from build123d import *

# Parameters (mm, degrees)
SKETCH_1_W           = 10
SKETCH_1_H           = 10
SKETCH_1_W_2         = 8
SKETCH_1_H_2         = 8
EXTRUDE_1_DEPTH      = 106.066
SKETCH_2_R           = 1
CUT_EXTRUDE_1_DEPTH  = 10
EXTRUDE_START        = -22
EXTRUDE_3_OUTLINE_R  = 1
EXTRUDE_3_DEPTH      = 34
EXTRUDE_7_DEPTH      = 15.36
EXTRUDE_7_DEPTH_BACK = 25.36
SKETCH_9_R           = 1
EXTRUDE_8_DEPTH      = 5
EXTRUDE_8_DEPTH_BACK = 15


# Read off the part's stored shape, not the designer's step: the extrude step
with BuildPart() as part:
    # Sketch 1 → Extrude 1 (new body)
    with BuildSketch(Plane.XY):
        with Locations((5, 5)):
            Rectangle(SKETCH_1_W, SKETCH_1_H)
        with Locations((5, 5)):
            Rectangle(SKETCH_1_W_2, SKETCH_1_H_2, mode=Mode.SUBTRACT)
    extrude(amount=EXTRUDE_1_DEPTH)

    # Sketch 2 → Cut-Extrude 1 (cut)
    with BuildSketch(Plane(origin=(10, 0, 0), x_dir=(0, 0, -1), z_dir=(1, 0, 0))):
        with Locations((-10, 5)):
            Circle(SKETCH_2_R)
    extrude(amount=-CUT_EXTRUDE_1_DEPTH, mode=Mode.SUBTRACT)

    # Extrude 3 outline → Extrude 3 (add)
    with BuildSketch(Plane(origin=(10, 0, 0), x_dir=(0, 0, -1), z_dir=(1, 0, 0)).offset(EXTRUDE_START)):
        with Locations((-10, 5)):
            Circle(EXTRUDE_3_OUTLINE_R)
    extrude(amount=EXTRUDE_3_DEPTH)

    # Sketch 9 → Extrude 7 (add, two sides: drawn at the far end of the back side and taken through both)
    with BuildSketch(Plane(origin=(10, 0, 0), x_dir=(0, 0, -1), z_dir=(1, 0, 0)).offset(-EXTRUDE_7_DEPTH_BACK)):
        with Locations(Location((-96.066, 5, 0), (0, 0, 270))):
            Circle(SKETCH_9_R)
    extrude(amount=EXTRUDE_7_DEPTH + EXTRUDE_7_DEPTH_BACK)

    # Sketch 10 → Extrude 8 (add, two sides: drawn at the far end of the back side and taken through both)
    with BuildSketch(Plane(origin=(10, 0, 0), x_dir=(0, 0, -1), z_dir=(1, 0, 0)).offset(-EXTRUDE_8_DEPTH_BACK)):
        with BuildLine():
            ThreePointArc((-96.556592177, 5.871389302), (-96.319584994, 5.967313109), (-96.066, 6))
            Line((-96.066, 6), (-96.066, 7.038352927))
            Line((-96.066, 7.038352927), (-97.733407302, 10))
            Line((-97.733407302, 10), (-98.881, 10))
            Line((-98.881, 10), (-96.556592177, 5.871389302))
        make_face()
        with BuildLine():
            Line((-96.066, 7.038352927), (-96.066, 6))
            ThreePointArc((-96.066, 6), (-95.56131799, 5.863305316), (-95.194610676, 5.490592137))
            Line((-95.194610676, 5.490592137), (-96.066, 7.038352927))
        make_face()
        with BuildLine():
            Line((-96.066, 6), (-96.066, 5))
            Line((-96.066, 5), (-95.575407823, 4.128610698))
            ThreePointArc((-95.575407823, 4.128610698), (-95.202694672, 4.49531801), (-95.066, 5))
            ThreePointArc((-95.066, 5), (-95.098686885, 5.253584971), (-95.194610676, 5.490592137))
            ThreePointArc((-95.194610676, 5.490592137), (-95.56131799, 5.863305316), (-96.066, 6))
        make_face()
        with BuildLine():
            Line((-96.556592177, 5.871389302), (-96.066, 5))
            Line((-96.066, 5), (-96.066, 6))
            ThreePointArc((-96.066, 6), (-96.319584994, 5.967313109), (-96.556592177, 5.871389302))
        make_face()
        with BuildLine():
            ThreePointArc((-95.066, 5), (-95.202694672, 4.49531801), (-95.575407823, 4.128610698))
            Line((-95.575407823, 4.128610698), (-93.251, 0))
            Line((-93.251, 0), (-92.379610698, 0.490592177))
            Line((-92.379610698, 0.490592177), (-95.194610676, 5.490592137))
            ThreePointArc((-95.194610676, 5.490592137), (-95.098686885, 5.253584971), (-95.066, 5))
        make_face()
        Polygon((-92.379610698, 0.490592177), (-93.251, 0), (-92.103407302, 0), align=None)
    extrude(amount=EXTRUDE_8_DEPTH + EXTRUDE_8_DEPTH_BACK)


solid = part.part
Work out the finished part from the listing and answer in its coordinate system (mm). A direction names the side the tool comes from. Coordinates: 2 decimals unless noted, no trailing zeros. Loops run counter-clockwise (first coordinate to the right, second up) from the corner with the lowest first, then second, coordinate; pieces in that order, holes last. Notation, with made-up numbers: (26.25, 37) -> (79.25, 37) arc R16 ccw to (79.25, 65) -> close; hole circle Ø2 at (4, 58). An arc over 180 degrees is marked (long way). Write each question's results on one line, items separated by ' | '. Start each with the question number.
1) Consider line 1 along X through (y, z) = (5.25, 92); line 2 along Z through (x, y) = (5, 7). Determine where each line is inside the solid, lowest interval first.
2) Flat-ended cylindrical pins translate along their axes: P1, Ø5, axis at y = 6.5, z = 34, coming from the +X side; P2, Ø6, axis at x = 14.5, y = 1.5, coming from the +Z side; P3, Ø12, axis at x = 20, z = 35.5, coming from the -Y side; P4, Ø3, axis at y = 2.5, z = 94.5, coming from the -X side. Find the tip coordinate at first contact, or state that the pin passes through.
3) The mould has two halves that part along X. Classify faces 1 (the cylindrical face through (-9.494, 4.539, 96.953)), 2 (the flat face through (22, 5, 10)), 3 (the flat face through (5, 9, 102)): pulls with the +X half, pulls with the -X half, needs draft (parallel to the pull), parting line crosses it, or undercut.
4) Find section C-C on z = 10. Determine the outline of the cut face in (x, y).
5) Find section D-D on x = 4.5. Determine the outline of the cut face in (y, z), then the cut area to 3 significant figures.
6) Find section B-B on z = 86. Determine the outline of the cut face in (x, y), then the cut area to 3 significant figures.
7) For faces 4 (the cylindrical face through (19.279, 4.539, 96.953)), 5 (the flat face through (9, 5, 48)), 6 (the flat face through (5, 9, 48)), determine the directions among +Z, -Z, +X, -X, +Y, -Y from which every point of the face is accessible in a straight line to the end or side of a thin tool.
8) Find section A-A on x = 12. Determine the outline of the cut face in (y, z).
Response values:
1) line 1: x = 0 to 1, 9 to 10 | line 2: z = 96.04 to 97.19
2) P1: stops at x = 10 | P2: stops at z = 96.93 | P3: passes through | P4: stops at x = -5
3) face 1: needs draft | face 2: pulls with the +X half | face 3: undercut
4) outline: (-12, 4) -> (0, 4) -> (0, 0) -> (10, 0) -> (10, 4) -> (22, 4) -> (22, 6) -> (10, 6) -> (10, 10) -> (0, 10) -> (0, 6) -> (-12, 6) -> close; hole (1, 1) -> (9, 1) -> (9, 4) -> (1, 4) -> close; hole (1, 6) -> (9, 6) -> (9, 9) -> (1, 9) -> close
5) outline: (0, 0) -> (1, 0) -> (1, 92.67) -> (9, 97.17) -> (9, 0) -> (10, 0) -> (10, 106.07) -> (9, 106.07) -> (9, 98.32) -> (5.87, 96.56) arc R1 ccw to (4.13, 95.58) -> (1, 93.81) -> (1, 106.07) -> (0, 106.07) -> close; circle Ø2 at (5, 10) | area: 226 mm^2
6) outline: (0, 0) -> (10, 0) -> (10, 10) -> (0, 10) -> close; hole (1, 1) -> (9, 1) -> (9, 9) -> (1, 9) -> close | area: 36.0 mm^2
7) face 4: +X | face 5: none | face 6: -Z
8) outline: (0, 92.1) -> (10, 97.73) -> (10, 98.88) -> (5.87, 96.56) arc R1 ccw to (4.13, 95.58) -> (0, 93.25) -> close; circle Ø2 at (5, 10)
